Work out the finished part from the listing and answer in its coordinate system (mm). Face numbers are marked on the shaded views. Give positions to 0.01 mm unless a question says otherwise; leave off trailing zeros. Write each loop counter-clockwise with the first axis right and the second up, starting at its lowest first coordinate (ties: lowest second). Pieces come first, ordered by that corner, then holes. Notation, with made-up numbers: (21, 26) -> (78, 26) arc R10 ccw to (78, 34) -> close; hole circle Ø1 at (-12, 23). An arc over 180 degrees is marked (long way). Use a Markdown table: item, result. Add a question column.
Q1. For a pull along Y with two mould halves and no side action, classify the marked faces 1, 2 and 3 as pulls with the +Y half, pulls with the -Y half, needs draft (parallel to the pull), parting line crosses it, or undercut.
Q2. Consider line 1 (Y direction, x = -10.5, z = 0); line 2 (X direction, y = -2.25, z = 4.5). Determine where each line is inside the solid, lowest interval first.
Q3. Section B-B, the plane z = 5.25 is taken. Give the vertices of the cut face in (x, y).
Q4. Section A-A, the plane x = -10.25 is taken. Give the vertices of the cut face in (y, z), plus the area to 3 significant figures.
Q5. Each of these flat-tipped pins is pushed along its axis until it touches: pin 1 Ø3 at (x, z) = (-5.5, 0) entering from +Y; pin 2 Ø4 at (x, z) = (-8, -2.5) entering from -Y; pin 3 Ø1 at (x, y) = (-2, 3.5) entering from +Z. Where does it stop, or does it pass through?
Q6. Section C-C, the plane y = -5 is taken. Give the vertices of the cut face in (x, z).
from build123d import *

# Parameters (mm, degrees)
F2_R     = 1
F3_R     = 2.25
F4_DEPTH = 7


with BuildPart() as f1:
    # F0 (on Front) → F1 (revolve)
    with BuildSketch(Plane.XZ):
        with BuildLine():
            Line((-14.220479, 0), (0, 0))
            Line((0, 0), (0, 6))
            Line((0, 6), (-2, 6))
            Line((-2, 6), (-2, 3.75))
            Line((-2, 3.75), (-11, 3.75))
            Line((-11, 3.75), (-12.236166, 3.75))
            ThreePointArc((-12.236166, 3.75), (-13.559041, 3.25), (-14.220479, 2))
            Line((-14.220479, 2), (-14.220479, 0))
        make_face()
    revolve(axis=Axis((-7.11024, 0, 0), (1, 0, 0)))

    # F2
    f2_edges = [f1.edges().sort_by_distance(p)[0] for p in [
        (-2, 0, -3.75),
    ]]
    fillet(f2_edges, radius=F2_R)

    # F3 (on face) → F4 (cut)
    with BuildSketch(Plane(origin=(-14.220479, 0, 0), x_dir=(0, -1, 0), z_dir=(-1, 0, 0))):
        Circle(F3_R)
    extrude(amount=-F4_DEPTH, mode=Mode.SUBTRACT)


solid = f1.part
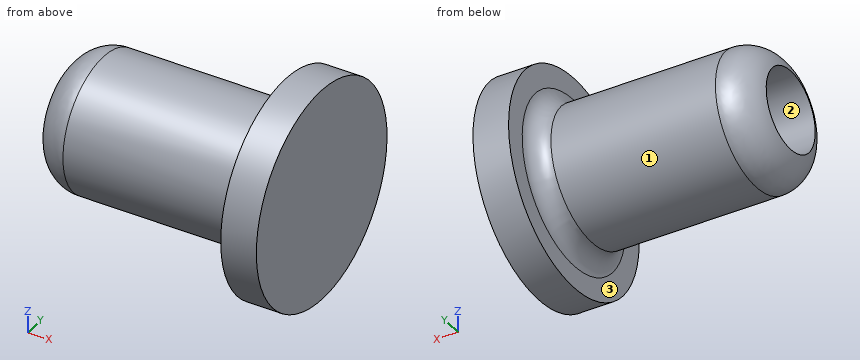
Result set:
| question | item | result |
|---|---|---|
| 1 | face 1 | parting line crosses it |
| 1 | face 2 | undercut |
| 1 | face 3 | needs draft |
| 2 | line 1 | y = -3.75 to -2.25, 2.25 to 3.75 |
| 2 | line 2 | x = -2 to 0 |
| 3 | outline | (-2, -2.9) -> (0, -2.9) -> (0, 2.9) -> (-2, 2.9) -> close |
| 4 | outline | circle Ø7.5 at (0, 0); hole circle Ø4.5 at (0, 0) |
| 4 | area | 28.3 mm2 |
| 5 | pin 1 | stops at y = 3.75 |
| 5 | pin 2 | stops at y = -3.72 |
| 5 | pin 3 | stops at z = 5.2 |
| 6 | outline | (-2, -3.32) -> (0, -3.32) -> (0, 3.32) -> (-2, 3.32) -> close |
